Could you check a few things on this drawing? It's one solid part, dimensions in mm from its lowest x, y, z. Coordinates: 2 decimals unless noted, no trailing zeros. Order: outer loops, then holes, each group sorted by start corner. A loop starts at its lowest first (then second) coordinate and runs counter-clockwise, first axis right, second up.
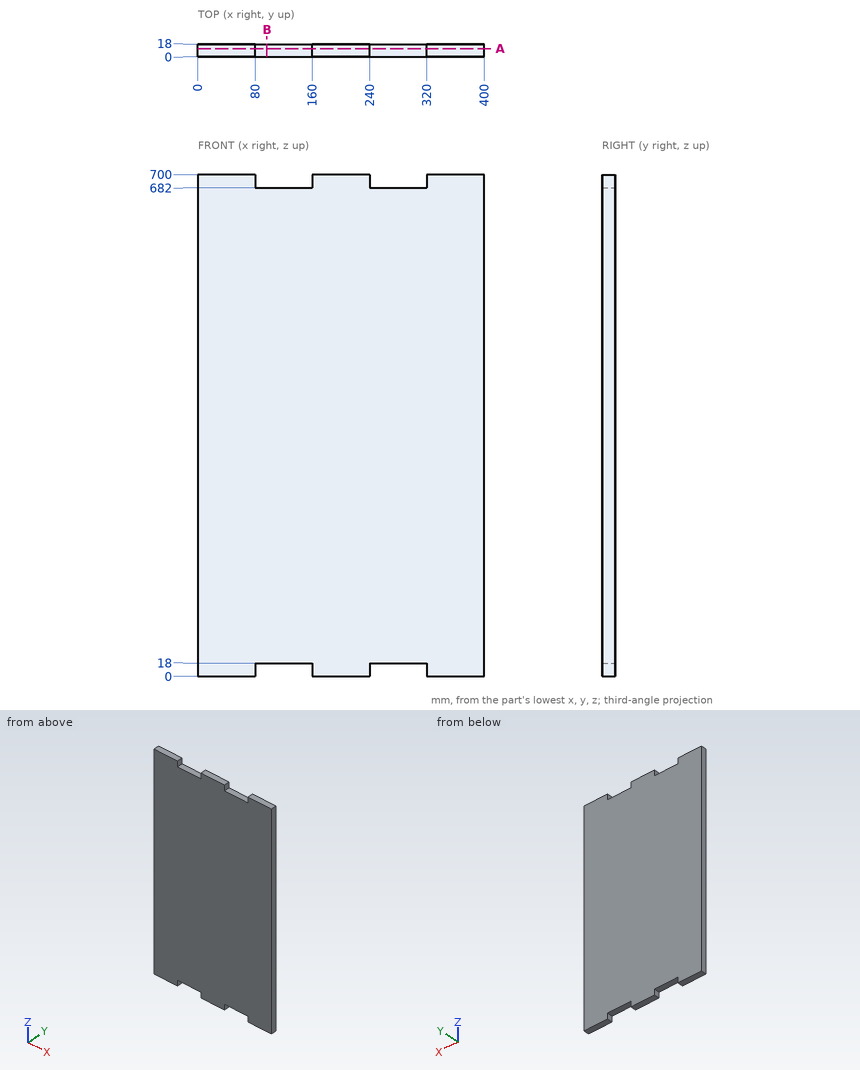
Item 1: I need wall thicknesses on line 1 (Z direction, x = 254, y = 3). Which ranges of the line are inside material? Lowest first, please.
Item 2: Suppose I cut it at B-B (x = 96.5). List the corners of the cut face in (y, z) for me, and give its area (3 significant figures).
Item 3: For pin 1 Ø5.5 at (x, y) = (289, 7.5) entering from +Z, with a flat end and sliding along its axis, tell me the tip position at first contact or that it passes through.
Item 4: Suppose I cut it at A-A (y = 11.5). List the corners of the cut face in (x, z) for me, and give its area (3 significant figures).
Geometry results:
1. line 1: z = 18 to 682
2. outline: (0, 18) - (18, 18) - (18, 682) - (0, 682) - close
2. area: 12,000 mm2
3. pin 1: stops at z = 682
4. outline: (0, 0) - (80, 0) - (80, 18) - (160, 18) - (160, 0) - (240, 0) - (240, 18) - (320, 18) - (320, 0) - (400, 0) - (400, 700) - (320, 700) - (320, 682) - (240, 682) - (240, 700) - (160, 700) - (160, 682) - (80, 682) - (80, 700) - (0, 700) - close
4. area: 274,000 mm2
